from build123d import *

# Parameters (mm, degrees)
SKETCH1_R           = 1
BOSS_EXTRUDE1_DEPTH = 16
CUT_EXTRUDE1_START  = 8
SKETCH4_R           = 0.5
SKETCH4_R_2         = 1
CUT_EXTRUDE1_DEPTH  = 8
FILLET1_R           = 10


with BuildPart() as part:
    # Sketch1 → Boss-Extrude1 (new body)
    with BuildSketch(Plane.XY):
        with BuildLine():
            ThreePointArc((0, 20), (-0.37218717, 23.088420816), (-1.467437405, 26))
            Line((-1.467437405, 26), (-3.726208596, 23.741228809))
            ThreePointArc((-3.726208596, 23.741228809), (-3.183230826, 21.90552958), (-3, 20))
            Line((-3, 20), (-3, 0))
            ThreePointArc((-3, 0), (-1.5, -1.5), (0, 0))
            Line((0, 0), (0, 20))
        make_face()
        with Locations((-1.5, 0)):
            Circle(SKETCH1_R, mode=Mode.SUBTRACT)
    extrude(amount=BOSS_EXTRUDE1_DEPTH)

    # Sketch4 → Cut-Extrude1 (cut)
    # profile 1 of 10: a face of its own
    with BuildSketch(Plane(origin=(0, 0, 12), x_dir=(-1, 0, 0), z_dir=(0, 0, -1)).offset(CUT_EXTRUDE1_START)):
        with Locations((1.5, 1.5)):
            Circle(SKETCH4_R)
    # profile 2 of 10: a face of its own
    with BuildSketch(Plane(origin=(0, 0, 12), x_dir=(-1, 0, 0), z_dir=(0, 0, -1)).offset(CUT_EXTRUDE1_START)):
        with BuildLine():
            ThreePointArc((3, 0), (1.5, 1.5), (0, 0))
            ThreePointArc((0, 0), (1.5, -1.5), (3, 0))
        make_face()
        with Locations((1.5, 0)):
            Circle(SKETCH4_R_2, mode=Mode.SUBTRACT)
    # profile 3 of 10: a face of its own
    with BuildSketch(Plane(origin=(0, 0, 12), x_dir=(-1, 0, 0), z_dir=(0, 0, -1)).offset(CUT_EXTRUDE1_START)):
        with BuildLine():
            ThreePointArc((1.993006649, 1.416666667), (2.722601728, 0.869048338), (3, 0))
            Line((3, 0), (3, 1.5))
            Line((3, 1.5), (2, 1.5))
            ThreePointArc((2, 1.5), (1.998248595, 1.45818687), (1.993006649, 1.416666667))
        make_face()
    # profile 4 of 10: a face of its own
    with BuildSketch(Plane(origin=(0, 0, 12), x_dir=(-1, 0, 0), z_dir=(0, 0, -1)).offset(CUT_EXTRUDE1_START)):
        with BuildLine():
            ThreePointArc((1.5, 1.5), (1.25, 1.479019946), (1.006993351, 1.416666667))
            ThreePointArc((1.006993351, 1.416666667), (1.177251388, 1.118118692), (1.5, 1))
            ThreePointArc((1.5, 1), (1.822748612, 1.118118692), (1.993006649, 1.416666667))
            ThreePointArc((1.993006649, 1.416666667), (1.75, 1.479019946), (1.5, 1.5))
        make_face()
    # profile 5 of 10: a face of its own
    with BuildSketch(Plane(origin=(0, 0, 12), x_dir=(-1, 0, 0), z_dir=(0, 0, -1)).offset(CUT_EXTRUDE1_START)):
        with BuildLine():
            Line((0, 1.5), (0, 0))
            ThreePointArc((0, 0), (0.277398272, 0.869048338), (1.006993351, 1.416666667))
            ThreePointArc((1.006993351, 1.416666667), (1.001751405, 1.45818687), (1, 1.5))
            Line((1, 1.5), (0, 1.5))
        make_face()
    # profile 6 of 10: a face of its own
    with BuildSketch(Plane(origin=(0, 0, 12), x_dir=(-1, 0, 0), z_dir=(0, 0, -1)).offset(CUT_EXTRUDE1_START)):
        with BuildLine():
            ThreePointArc((1, 1.5), (1.001751405, 1.45818687), (1.006993351, 1.416666667))
            ThreePointArc((1.006993351, 1.416666667), (1.25, 1.479019946), (1.5, 1.5))
            Line((1.5, 1.5), (1, 1.5))
        make_face()
    # profile 7 of 10: a face of its own
    with BuildSketch(Plane(origin=(0, 0, 12), x_dir=(-1, 0, 0), z_dir=(0, 0, -1)).offset(CUT_EXTRUDE1_START)):
        with BuildLine():
            ThreePointArc((1.5, 1.5), (1.75, 1.479019946), (1.993006649, 1.416666667))
            ThreePointArc((1.993006649, 1.416666667), (1.998248595, 1.45818687), (2, 1.5))
            Line((2, 1.5), (1.5, 1.5))
        make_face()
    # profile 8 of 10: a face of its own
    with BuildSketch(Plane(origin=(0, 0, 12), x_dir=(-1, 0, 0), z_dir=(0, 0, -1)).offset(CUT_EXTRUDE1_START)):
        with BuildLine():
            ThreePointArc((2, 1.5), (1.5, 2), (1, 1.5))
            Line((1, 1.5), (1.5, 1.5))
            Line((1.5, 1.5), (2, 1.5))
        make_face()
    # profile 9 of 10: a face of its own
    with BuildSketch(Plane(origin=(0, 0, 12), x_dir=(-1, 0, 0), z_dir=(0, 0, -1)).offset(CUT_EXTRUDE1_START)):
        with BuildLine():
            ThreePointArc((1, 1.5), (1.001751405, 1.45818687), (1.006993351, 1.416666667))
            ThreePointArc((1.006993351, 1.416666667), (1.25, 1.479019946), (1.5, 1.5))
            Line((1.5, 1.5), (1, 1.5))
        make_face()
    # profile 10 of 10: a face of its own
    with BuildSketch(Plane(origin=(0, 0, 12), x_dir=(-1, 0, 0), z_dir=(0, 0, -1)).offset(CUT_EXTRUDE1_START)):
        with BuildLine():
            ThreePointArc((1.5, 1.5), (1.75, 1.479019946), (1.993006649, 1.416666667))
            ThreePointArc((1.993006649, 1.416666667), (1.998248595, 1.45818687), (2, 1.5))
            Line((2, 1.5), (1.5, 1.5))
        make_face()
    extrude(amount=-CUT_EXTRUDE1_DEPTH, mode=Mode.SUBTRACT)

    # Fillet1
    # the kernel refuses this fillet: 10 mm, written as the material it takes off along each edge
    with BuildSketch(Plane(origin=(-2, 1.5, 4), x_dir=(-1, 0, 0), z_dir=(0, 0, 1))) as fillet1_piece_1:
        with BuildLine():
            CenterArc((3.666666667, -9.637888197), FILLET1_R, 105.466009953, 7.913858162)
            Line((-0.301587302, -0.458947057), (-0.380952381, -0.275368234))
            ThreePointArc((-0.380952381, -0.275368234), (-0.249286732, -0.164750894), (-0.2, 0))
            Line((-0.2, 0), (0, 0.2))
            ThreePointArc((0, 0.2), (0.5, 0.2), (0.946666667, 0.192757764))
            Line((0.946666667, 0.192757764), (1, 0))
        make_face()
    extrude(amount=8, mode=Mode.SUBTRACT)
    with BuildSketch(Plane(origin=(-1, 1.5, 4), x_dir=(-0.5491696473652747, 0.8357108940373459, 0), z_dir=(0, 0, 1))) as fillet1_piece_2:
        with BuildLine():
            CenterArc((6.040866121, -8.35710894), FILLET1_R, 123.310065942, 7.913858162)
            Line((-0.549169647, -0.835710894), (-0.680970363, -0.685282933))
            ThreePointArc((-0.680970363, -0.685282933), (-0.441727002, -0.308021518), (-0.167142179, 0.109833929))
            Line((-0.167142179, 0.109833929), (0.109833929, 0.167142179))
            ThreePointArc((0.109833929, 0.167142179), (0.274584824, 0.117855447), (0.439335718, 0.167142179))
            Line((0.439335718, 0.167142179), (0.549169647, 0))
        make_face()
    extrude(amount=8, mode=Mode.SUBTRACT)


solid = part.part
Source: CAD feature listing. Evaluate the final solid. Frame: model axes, mm. A direction names the side the tool comes from. Give positions to 0.01 mm unless a question says otherwise; leave off trailing zeros. Write each loop counter-clockwise with the first axis right and the second up, starting at its lowest first coordinate (ties: lowest second). Pieces come first, ordered by that corner, then holes. Notation, with made-up numbers: (-17, 40) - (10, 40) arc R15 cw to (10, 61) - close; hole circle Ø8 at (-16, 44). An arc over 180 degrees is marked (long way). Write item = value, one per line. Start each with the question number.
Q1. Cut plane C-C, the plane y = 18. Return loops of the section in (x, z).
Q2. Cut plane B-B, the plane z = 6.5. Return loops of the section in (x, y).
Q3. Reachability of faces 5 (the flat face through (-1, 12, 16)), 6 (the cylindrical face through (-0.67, 1.71, 7.94)), 7 (the flat face through (-3, 10, 8)) from +Z, -Z, +X, -X, +Y, -Y: full face, straight path, thin tool, end or side. Return the list, or none.
Q4. Draft query along Y for faces 1 (the cylindrical face through (-1.717, -0.976, 1.972)), 2 (the flat face through (-1.1, 1.1, 12)), 3 (the cylindrical face through (-1.717, -0.976, 13.972)), 4 (the cylindrical face through (-1.5, -1.5, 2)). Return one class per face: +Y half, -Y half, draft (parallel to the pull), parting line (faces both ways), or undercut.
Q5. Cut plane A-A, the plane z = 1.5. Return loops of the section in (x, y).
Q6. Pin query (flat end, axial travel): pin 1 Ø1.6 at (x, y) = (-1.5, 0) entering from -Z; pin 2 Ø1 at (y, z) = (3, 11.5) entering from -X. Return the tip coordinate at first contact, or that it passes through.
Q7. Material intervals for probe 1 along Z at (x, y) = (-0.5, 1); probe 2 along X at (y, z) = (0, 1.15); probe 3 along Y at (x, z) = (-1.25, 12.5), sorted ascending.
Computed values:
q1.outline = (-3, 0) - (0, 0) - (0, 16) - (-3, 16) - close
q2.outline = (-3.73, 23.74) arc R10 cw to (-3, 20) - (-3, 1.5) arc R10 ccw to (-1.7, 1.96) arc R0.5 cw to (-1.3, 1.96) arc R10 ccw to (0, 1.5) - (0, 20) arc R13 ccw to (-1.47, 26) - close
q3.face_5 = +Z, +X, -X, +Y, -Y
q3.face_6 = -Y
q3.face_7 = +Z, -Z, -X, -Y
q4.face_1 = undercut
q4.face_2 = draft
q4.face_3 = undercut
q4.face_4 = -Y half
q5.outline = (-3.73, 23.74) arc R10 cw to (-3, 20) - (-3, 0) arc R1.5 ccw to (0, 0) - (0, 20) arc R13 ccw to (-1.47, 26) - close; hole circle Ø2 at (-1.5, 0)
q6.pin_1 = through
q6.pin_2 = -3
q7.probe_1 = 0 to 4, 12 to 16
q7.probe_2 = -3 to -2.5, -0.5 to 0
q7.probe_3 = -1.48 to -0.97, 0.97 to 25.56
